Can you work these out from the drawing? Everything is in mm from the part's minimum corner. Give positions to 0.01 mm unless a question says otherwise; leave off trailing zeros. Order: outer loops, then holes, each group sorted by start corner. A loop starts at its lowest first (then second) coordinate and runs counter-clockwise, first axis right, second up. Notation, with made-up numbers: M 57.5,82.5 L 108.5,82.5 A17 cw 108.5,113.5 Z; hole C 35.5,11 d3. An arc over 180 degrees is marked long. Answer as a JSON object with one key per item and string values.
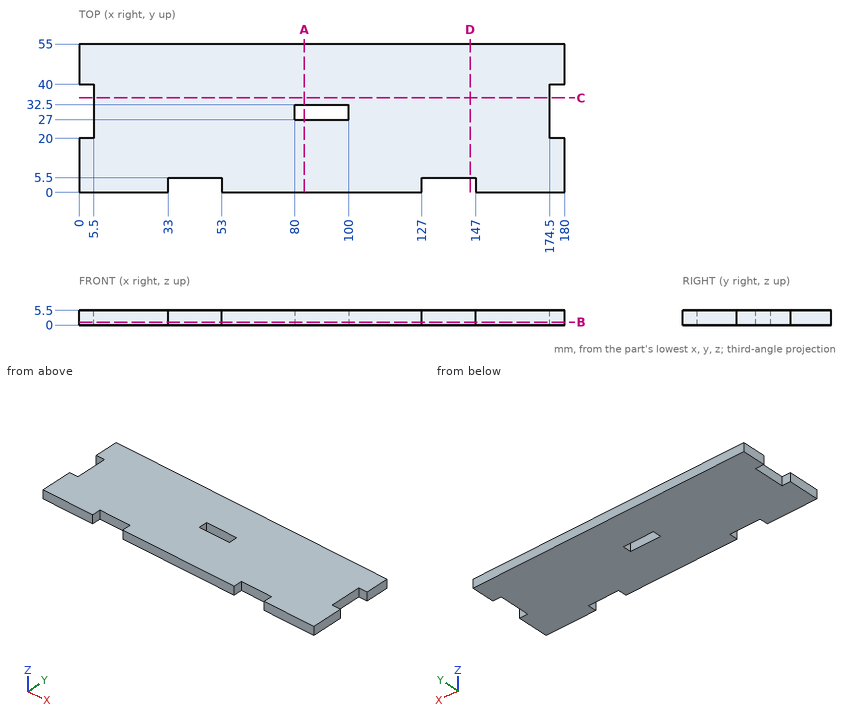
1) I need wall thicknesses on L1, parallel to X at y = 5, z = 1; L2, parallel to Y at x = 49.5, z = 0.9; L3, parallel to X at y = 24.5, z = 1.25. Which ranges of each line are inside material? Lowest first, please.
Results found:
{"L1": "x = 0 to 33, 53 to 127, 147 to 180", "L2": "y = 5.5 to 55", "L3": "x = 5.5 to 174.5"}
2) I want a section at A-A on x = 83.5. Write out the boundary of the cut face in (y, z).
Results found:
{"outline": "M 0,0 L 27,0 L 27,5.5 L 0,5.5 Z; M 32.5,0 L 55,0 L 55,5.5 L 32.5,5.5 Z"}
3) I'm going to push a flat-ended pin straight in: pin 1 Ø1.6 at (y, z) = (26, 1.5) entering from +X. Where does the tip first touch, or does it pass through?
Results found:
{"pin 1": "stops at x = 174.5"}
4) I want a section at C-C on y = 35. Write out the boundary of the cut face in (x, z), and give its area (4 significant figures).
Results found:
{"outline": "M 5.5,0 L 174.5,0 L 174.5,5.5 L 5.5,5.5 Z", "area": "929.5 mm²"}
5) I want a section at B-B on z = 1.1. Write out the boundary of the cut face in (x, y), and give its area (3 significant figures).
Results found:
{"outline": "M 0,0 L 33,0 L 33,5.5 L 53,5.5 L 53,0 L 127,0 L 127,5.5 L 147,5.5 L 147,0 L 180,0 L 180,20 L 174.5,20 L 174.5,40 L 180,40 L 180,55 L 0,55 L 0,40 L 5.5,40 L 5.5,20 L 0,20 Z; hole M 80,27 L 100,27 L 100,32.5 L 80,32.5 Z", "area": "9,350 mm²"}
6) I want a section at D-D on x = 145. Write out the boundary of the cut face in (y, z).
Results found:
{"outline": "M 5.5,0 L 55,0 L 55,5.5 L 5.5,5.5 Z"}
